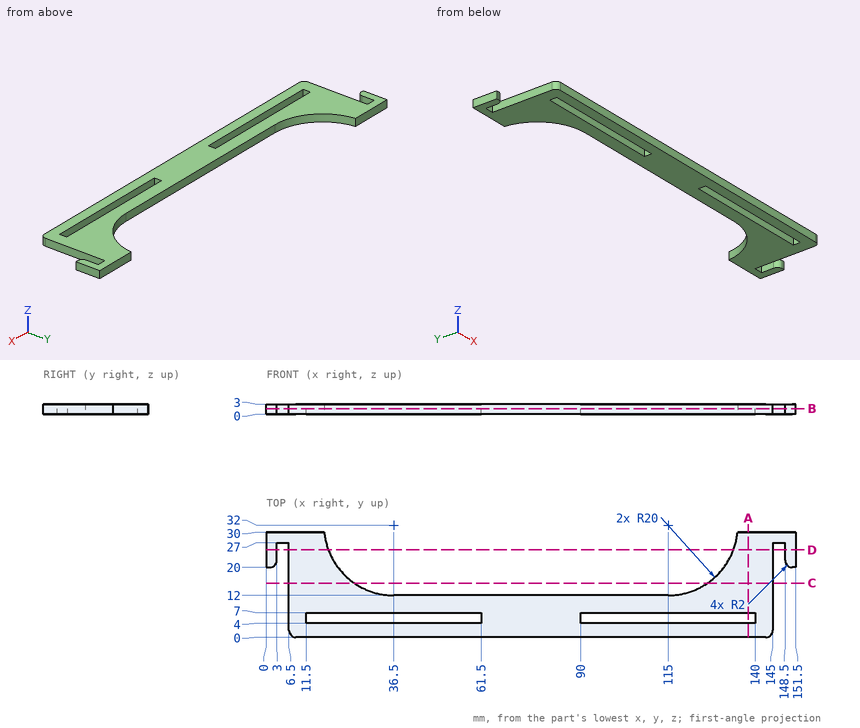
Here's the drawing with two shaded views (mm, measured from the low corner). I have some questions. Give positions to 0.01 mm unless a question says otherwise; leave off trailing zeros. Order: outer loops, then holes, each group sorted by start corner. A loop starts at its lowest first (then second) coordinate and runs counter-clockwise, first axis right, second up. Notation, with made-up numbers: M -27.5,-28.75 L 23.5,-28.75 A10 cw 23.5,-20.75 Z; hole C 66,-3 d3. An arc over 180 degrees is marked long. Answer as a JSON object with one key per item and string values. Group by question number.
1) Suppose I cut it at B-B, the plane z = 1.7. Write out the boundary of the cut face in (x, y), plus the area to 3 significant figures.
2) Suppose I cut it at A-A, the plane x = 138. Write out the boundary of the cut face in (y, z).
3) Suppose I cut it at D-D, the plane y = 25. Write out the boundary of the cut face in (x, z) (3 decimals).
4) Please list where these lines run through material, in increasing order: L1, parallel to X at y = 5, z = 2.2; L2, parallel to Y at x = 58, z = 2.7; L3, parallel to X at y = 25, z = 0.9 (3 decimals). Write a range as [from, to].
5) I'm going to push flat-ended pins straight in: pin 1 Ø1.5 at (y, z) = (9, 2) entering from -X; pin 2 Ø1.5 at (y, z) = (7, 2.5) entering from +X; pin 3 Ø1.5 at (x, z) = (47.5, 2) entering from +Y. Where does each tip first touch, or does it pass through?
6) Suppose I cut it at C-C, the plane y = 15.5. Write out the boundary of the cut face in (x, z).
Results found:
{
 "1": {"outline": "M 0,20 L 1,20 A2 ccw 3,22 L 3,27 L 6.5,27 L 6.5,2 A2 ccw 8.5,0 L 143,0 A2 ccw 145,2 L 145,27 L 148.5,27 L 148.5,22 A2 ccw 150.5,20 L 151.5,20 L 151.5,30 L 134.9,30 A20 cw 115,12 L 36.5,12 A20 cw 16.6,30 L 0,30 Z; hole M 11.5,4 L 61.5,4 L 61.5,7 L 11.5,7 Z; hole M 90,4 L 140,4 L 140,7 L 90,7 Z", "area": "1,970 mm²"},
 "2": {"outline": "M 0,0 L 4,0 L 4,3 L 0,3 Z; M 7,0 L 30,0 L 30,3 L 7,3 Z"},
 "3": {"outline": "M 0,0 L 3,0 L 3,3 L 0,3 Z; M 6.5,0 L 17.765,0 L 17.765,3 L 6.5,3 Z; M 133.735,0 L 145,0 L 145,3 L 133.735,3 Z; M 148.5,0 L 151.5,0 L 151.5,3 L 148.5,3 Z"},
 "4": {"L1": "[6.5, 11.5], [61.5, 90], [140, 145]", "L2": "[0, 4], [7, 12]", "L3": "[0, 3], [6.5, 17.765], [133.735, 145], [148.5, 151.5]"},
 "5": {"pin 1": "x = 6.5", "pin 2": "x = 145", "pin 3": "y = 12"},
 "6": {"outline": "M 6.5,0 L 25.2,0 L 25.2,3 L 6.5,3 Z; M 126.3,0 L 145,0 L 145,3 L 126.3,3 Z"}
}
